Autodesk Inventor part; units mm, degrees
ref_plane "YZ Plane" through (0, 0, 0) normal (1, 0, 0) x (0, 1, 0)
ref_plane "XZ Plane" through (0, 0, 0) normal (0, 1, 0) x (-1, 0, 0)
ref_plane "XY Plane" through (0, 0, 0) normal (0, 0, 1) x (1, 0, 0)
sketch "Sketch1" plane through (0, 0, 0) normal (0, 1, 0) x (-1, 0, 0)
  circle A0 centre (0, 0) radius 76.2
  dimension "d0" = 152.4
extrude "Extrusion1" add sketch "Sketch1" along normal blind 11.43
sketch "Sketch2" plane through (0, 11.43, 0) normal (0, 1, 0) x (1, 0, 0)
  circle A0 centre (0, 0) radius 76.2
  line L0 (0.1023, 76.1999) -> (0.1023, 63.4999) construction
  arc A1 (-8.3552, 59.1187) -> (8.4222, 58.8626) centre (0.1023, 63.4999) ccw
  line L1 (8.4222, 58.8626) -> (15.4584, 74.6155)
  line L2 (-8.3552, 59.1187) -> (-16.2911, 74.4382)
  dimension "d3" = 12.7
  dimension "d4" = 19.05
  dimension "d16" = 31.75
extrude "Extrusion2" cut sketch "Sketch2" against normal through all contours L1 A1 L2 A0 picked at (1.6562, 64.6745)
fillet "Fillet1" radius 9.525 1 edges at (-16.2911, 5.715, -74.4382)
fillet "Fillet2" radius 9.525 1 edges at (15.4584, 5.715, -74.6155)
pattern_circular "Circular Pattern1" count 5 over 360 about axis through (0, -10, 0) along (0, 1, 0) of "Extrusion2", "Fillet1", "Fillet2"
sketch "Sketch4" plane through (0, 0, 0) normal (0, -1, 0) x (1, 0, 0)
  circle A0 centre (0, 0) radius 3.175
  dimension "d19" = 6.35
hole "Hole1" at (0, 0, 0) direction (0, 1, 0) diameter 6.35 end through all
sketch "Sketch5" plane through (0, 0, 0) normal (0, -1, 0) x (1, 0, 0)
  circle A0 centre (0, -9.779) radius 1.9844
  circle A1 centre (0, 0) radius 3.175
  arc A2 (67.6814, -9.2124) -> (76.1994, 0.2962) centre (66.6745, 0.2592) ccw
  arc A3 (76.1994, 0.2962) -> (62.0688, 44.203) centre (0, 0) ccw
  arc A4 (62.0688, 44.203) -> (50.0431, 47.1934) centre (54.3102, 38.6777) ccw
  line L0 (50.0431, 47.1934) -> (41.5086, 42.9169)
  arc A5 (27.7848, 52.5712) -> (41.5086, 42.9169) centre (37.2415, 51.4327) ccw
  line L1 (27.7848, 52.5712) -> (29.6763, 61.522)
  arc A6 (29.6763, 61.522) -> (23.2652, 72.5615) centre (20.357, 63.4913) ccw
  arc A7 (23.2652, 72.5615) -> (-22.8593, 72.6904) centre (0, 0) ccw
  arc A8 (-22.8593, 72.6904) -> (-29.4194, 62.1774) centre (-20.0019, 63.6041) ccw
  line L2 (-29.4194, 62.1774) -> (-27.9896, 52.7391)
  arc A9 (-41.4122, 42.6704) -> (-27.9896, 52.7391) centre (-37.4071, 51.3124) ccw
  line L3 (-41.4122, 42.6704) -> (-49.3405, 47.2352)
  arc A10 (-49.3405, 47.2352) -> (-61.8207, 44.5493) centre (-54.0931, 38.9806) ccw
  arc A11 (-61.8207, 44.5493) -> (-76.1966, 0.7221) centre (0, 0) ccw
  arc A12 (-76.1966, 0.7221) -> (-68.2253, -8.7657) centre (-66.672, 0.6318) ccw
  line L4 (-68.2253, -8.7657) -> (-58.8071, -10.3224)
  arc A13 (-53.379, -26.1995) -> (-58.8071, -10.3224) centre (-60.3604, -19.7199) ccw
  line L5 (-53.379, -26.1995) -> (-60.1703, -32.3291)
  arc A14 (-60.1703, -32.3291) -> (-61.4725, -45.0285) centre (-53.7885, -39.4) ccw
  arc A15 (-61.4725, -45.0285) -> (-24.2328, -72.2441) centre (0, 0) ccw
  arc A16 (-24.2328, -72.2441) -> (-12.7461, -67.5948) centre (-21.2037, -63.2136) ccw
  line L6 (-12.7461, -67.5948) -> (-8.3552, -59.1187)
  arc A17 (8.4222, -58.8626) -> (-8.3552, -59.1187) centre (0.1023, -63.4999) ccw
  line L7 (8.4222, -58.8626) -> (12.1532, -67.2156)
  arc A18 (12.1532, -67.2156) -> (23.8286, -72.3784) centre (20.8501, -63.3311) ccw
  arc A19 (23.8286, -72.3784) -> (61.2199, -45.3714) centre (0, 0) ccw
  arc A20 (61.2199, -45.3714) -> (60.3477, -33.0102) centre (53.5674, -39.7) ccw
  line L8 (60.3477, -33.0102) -> (53.6433, -26.215)
  arc A21 (58.5842, -10.1795) -> (53.6433, -26.215) centre (60.4236, -19.5253) ccw
  line L9 (58.5842, -10.1795) -> (67.6814, -9.2124)
  circle A22 centre (0, 0) radius 3.175
  circle A23 centre (0, 0) radius 3.175
  circle A24 centre (0, 0) radius 3.175
  circle A25 centre (9.779, 0) radius 1.9844
  circle A26 centre (0, 9.779) radius 1.9844
  circle A27 centre (-9.779, 0) radius 1.9844
  dimension "d27" = 9.779
  dimension "d28" = 3.9688
  dimension "d31" = 360
extrude "Extrusion3" cut sketch "Sketch5" against normal blind 12.7 contours A0 | A25 | A26 | A27
properties part number "gear wheel"
Model file for the job. Use its own axes, mm. A direction names the side the tool comes from. Round coordinates to 2 decimals unless told otherwise and drop trailing zeros. Loops run counter-clockwise (first coordinate to the right, second up) from the corner with the lowest first, then second, coordinate; pieces in that order, holes last. Notation, with made-up numbers: (-7, 54.5) -> (29, 54.5) arc R24 ccw to (29, 77.5) -> close; hole circle Ø6 at (70, 28). An arc over 180 degrees is marked (long way). Answer as CSV lines item,"result". Start each with the question number.
1) Slice it at D-D (x = -47.5). List the corners of the cut face in (y, z), plus the area to 3 significant figures.
2) Slice it at C-C (z = -36.5). List the corners of the cut face in (x, y).
3) Probe line 1 along Z through (x, y) = (0, 7.5) (3 decimals); line 2 along X through (y, z) = (3.5, 46.5); line 3 along Z through (x, y) = (11.5, 10.75). List the from-to ranges inside material, lowest first.
4) Slice it at B-B (y = 4). State how many separate pieces and enclosed holes the cut face has, plus the area to 3 significant figures.
5) Slice it at A-A (x = 0). List the corners of the cut face in (y, z) (3 decimals), plus the area to 3 significant figures.
6) Mould opens along X. For faces 5 (the face through (1, 11.43, -14)), 6 (the face through (31.88, 5.8, 43.56)), 7 (the face through (72.636, 5.635, 23.032)) say: +X half, -X half, draft (parallel to the pull), parting line (faces both ways), or undercut.
7) Tool access for faces 1 (the face through (-45.32, 5.8, 44.92)), 2 (the face through (-28.695, 5.795, 57.392)), 3 (the face through (-0.19, 5.8, -53.98)), 4 (the face through (28.717, 5.795, 56.984)): list every direction of +Z, -Z, +X, -X, +Y, -Y with a clear straight run to the whole face (end or side of a thin tool).
8) Pin check, flat tips, straight feed: P1, Ø3.5, axis at x = 0, z = -9.779, coming from the +Y side; P2, Ø1.5, axis at x = -41.5, y = 6, coming from the -Z side; P3, Ø1.5, axis at y = 9.5, z = -37, coming from the -X side; P4, Ø5, axis at x = 2.5, y = 1.5, coming from the -Z side. Stop position of each tip, or through.
Filled in:
1,outline,"(0, -59.58) -> (11.43, -59.58) -> (11.43, 46.18) -> (0, 46.18) -> close"
1,area,"1,210 mm2"
2,outline,"(-62.86, 0) -> (62.54, 0) -> (62.54, 11.43) -> (-62.86, 11.43) -> close"
3,line 1,"z = -53.976 to -11.763, -7.795 to -3.175, 3.175 to 7.795, 11.763 to 76.2"
3,line 2,"x = -59.94 to -48.06, -29.19 to 29.09, 48.66 to 59.74"
3,line 3,"z = -65.75 to -0.99, 0.99 to 75.33"
4,separate pieces,"1"
4,enclosed holes,"5"
4,area,"15,700 mm2"
5,outline,"(0, -53.976) -> (11.43, -53.976) -> (11.43, -11.763) -> (0, -11.763) -> close; (0, -7.795) -> (11.43, -7.795) -> (11.43, -3.175) -> (0, -3.175) -> close; (0, 3.175) -> (11.43, 3.175) -> (11.43, 7.795) -> (0, 7.795) -> close; (0, 11.763) -> (11.43, 11.763) -> (11.43, 76.2) -> (0, 76.2) -> close"
5,area,"1,320 mm2"
6,face 5,"draft"
6,face 6,"undercut"
6,face 7,"+X half"
7,face 1,"+Z, +Y, -Y"
7,face 2,"-X, +Y, -Y"
7,face 3,"-Z, +Y, -Y"
7,face 4,"+X, +Y, -Y"
8,P1,"passes through"
8,P2,"stops at z = -64.39"
8,P3,"stops at x = -63.17"
8,P4,"stops at z = -55.33"
